Part model, mm, in its own coordinate system. Face numbers are marked on the shaded views. A direction names the side the tool comes from. Round coordinates to 2 decimals unless told otherwise and drop trailing zeros. Order: outer loops, then holes, each group sorted by start corner. A loop starts at its lowest first (then second) coordinate and runs counter-clockwise, first axis right, second up. Notation, with made-up numbers: (62, 50.5) - (87, 50.5) arc R22 ccw to (87, 58.5) - close; hole circle Ø7 at (87.5, 63.5). An arc over 180 degrees is marked (long way). Return JSON: item names as keys, results as strings. Group by question number.
Item 1: Saw through at B-B on x = -0.5. List the corners of the cut face in (y, z) (3 decimals).
Item 2: Two-plate mould, pull along X, no slides. Class the marked faces 3, 4 and 5: released by +X, released by -X, zero draft, split by the parting line, or undercut.
Item 3: Probe probe 1 along Y at (x, z) = (0, 1); probe 2 along Z at (x, y) = (-1.75, -0.5); probe 3 along X at (y, z) = (-0.5, 7.5) (3 decimals). List the from-to ranges inside material, lowest first.
Item 4: Tool access for the marked faces 1 and 2: list every direction of +Z, -Z, +X, -X, +Y, -Y with a clear straight run to the whole face (end or side of a thin tool).
Item 5: Drop a flat-ended pin along its axis: pin 1 (1.6 mm diameter, centred on x = -0.5, y = -4, fed in from -Z) (3 decimals). Give the stop position or say it passes through.
Item 6: Saw through at A-A on z = 2. List the corners of the cut face in (x, y) (1 decimal), and give its area (3 significant figures).
Item 7: Saw through at D-D on z = 5.25. List the corners of the cut face in (x, y) (3 decimals), and give its area (3 significant figures).
Item 8: Saw through at C-C on y = 5. List the corners of the cut face in (x, z) (3 decimals), and give its area (3 significant figures).
```python
from build123d import *

# Parameters (mm, degrees)
SKETCH1_W           = 6.35
SKETCH1_H           = 25.4
BOSS_EXTRUDE1_DEPTH = 3.175
BOSS_EXTRUDE2_DEPTH = 25.4
SKETCH3_R           = 1.5875
CUT_EXTRUDE1_DEPTH  = 3.175


with BuildPart() as part:
    # Sketch1 → Boss-Extrude1 (new body)
    with BuildSketch(Plane.XY):
        Rectangle(SKETCH1_W, SKETCH1_H)
    extrude(amount=BOSS_EXTRUDE1_DEPTH)

    # Sketch2 → Boss-Extrude2 (add)
    with BuildSketch(Plane(origin=(0, 12.7, 0), x_dir=(1, 0, 0), z_dir=(0, 1, 0))):
        Polygon((-3.175, -3.175), (-3.175, -8.503282658), (3.175, -3.175), align=None)
    extrude(amount=-BOSS_EXTRUDE2_DEPTH)

    # Sketch3 → Cut-Extrude1 (cut)
    with BuildSketch(Plane(origin=(0, 0, 0), x_dir=(-1, 0, 0), z_dir=(0, 0, -1))):
        with Locations((0, 4.233333333)):
            Circle(SKETCH3_R)
        with Locations((0, -4.233333333)):
            Circle(SKETCH3_R)
    extrude(amount=-CUT_EXTRUDE1_DEPTH, mode=Mode.SUBTRACT)


solid = part.part
```
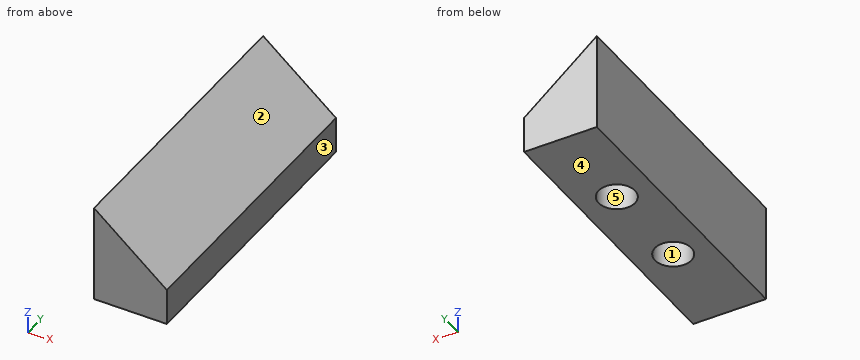
Filled in:
{
 "1": {"outline": "(-12.7, 0) - (-5.74, 0) - (-5.74, 3.175) - (-2.727, 3.175) - (-2.727, 0) - (2.727, 0) - (2.727, 3.175) - (5.74, 3.175) - (5.74, 0) - (12.7, 0) - (12.7, 6.259) - (-12.7, 6.259) - close"},
 "2": {"face 3": "released by +X", "face 4": "zero draft", "face 5": "undercut"},
 "3": {"probe 1": "y = -12.7 to -5.82, -2.65 to 2.65, 5.82 to 12.7", "probe 2": "z = 0 to 7.31", "probe 3": "x = -3.175 to -1.979"},
 "4": {"face 1": "-Z", "face 2": "+Z, +X, +Y, -Y"},
 "5": {"pin 1": "stops at z = 3.175"},
 "6": {"outline": "(-3.2, -12.7) - (3.2, -12.7) - (3.2, 12.7) - (-3.2, 12.7) - close; hole circle Ø3.2 at (0, -4.2); hole circle Ø3.2 at (0, 4.2)", "area": "145 mm^2"},
 "7": {"outline": "(-3.175, -12.7) - (0.702, -12.7) - (0.702, 12.7) - (-3.175, 12.7) - close", "area": "98.5 mm^2"},
 "8": {"outline": "(-3.175, 0) - (-1.39, 0) - (-1.39, 3.175) - (1.39, 3.175) - (1.39, 0) - (3.175, 0) - (3.175, 3.175) - (-3.175, 8.503) - close", "area": "28.3 mm^2"}
}
